```python
from build123d import *

# Parameters (mm, degrees)
F0_W     = 105.022209
F0_H     = 90.88391
F1_DEPTH = 92.202
F2_T     = -2.54
F3_W     = 99.942209
F3_H     = 87.122
F4_DEPTH = 2.794
F6_D     = 20.32
F6_DEPTH = 20.32
F7_R     = 6.310092
F8_DEPTH = 40.132


with BuildPart() as f1:
    # F0 (on Top) → F1 (new body)
    with BuildSketch(Plane.XY):
        with Locations((-23.505336, -22.022091)):
            Rectangle(F0_W, F0_H)
    extrude(amount=F1_DEPTH)

    # F2
    f2_openings = [f1.faces().sort_by_distance(p)[0] for p in [
        (-23.505337, -67.464046, 46.101),
    ]]
    offset(amount=F2_T, openings=f2_openings)

    # F3 (on face) → F4 (join)
    with BuildSketch(Plane.XZ.offset(67.464046)):
        with Locations((-23.505336, 46.101)):
            Rectangle(F3_W, F3_H)
    extrude(amount=-F4_DEPTH)

    # F6
    with Locations(Plane.XZ.offset(67.464046)):
        with Locations((-50.33106, 63.634276)):
            Hole(F6_D / 2, depth=F6_DEPTH)

    # F7 (on face) → F8 (join)
    with BuildSketch(Plane.XZ.offset(67.464046)):
        with Locations((-52.374396, 25.210666)):
            Circle(F7_R)
    extrude(amount=F8_DEPTH)


solid = f1.part
```
Source: CAD feature listing. Evaluate the final solid. Frame: model axes, mm. A direction names the side the tool comes from. Give positions to 0.01 mm unless a question says otherwise; leave off trailing zeros. Write each loop counter-clockwise with the first axis right and the second up, starting at its lowest first coordinate (ties: lowest second). Pieces come first, ordered by that corner, then holes. Notation, with made-up numbers: (38, 66.25) - (73, 66.25) arc R22 cw to (73, 89.25) - close; hole circle Ø11 at (-5, 64.25). An arc over 180 degrees is marked (long way). One line per item, written item: value. Start each with the question number.
Q1. Draft query along Z for faces 4 (the face through (-49.463, -87.249, 19.613)), 5 (the face through (-24, -21, 2.54)), 6 (the face through (-24, 23.42, 45)), 7 (the face through (-24, -64.67, 47)). Return one class per face: +Z half, -Z half, draft (parallel to the pull), parting line (faces both ways), or undercut.
Q2. Section query B-B, the plane y = -16.5. Return the cut outline in (x, z).
Q3. Set-up query: faces 1 (the face through (-73.476, -22, 45)), 2 (the face through (-48.129, -66.047, 53.716)), 3 (the face through (29.006, -23, 45)). Return all of +Z, -Z, +X, -X, +Y, -Y with unobstructed straight access to the full face (end or side cutting, diameter ignored); none if empty.
Q4. First-contact query: pin 1 Ø2 at (x, z) = (-10.5, 38.5) entering from -Y; pin 2 Ø1.5 at (x, y) = (-43, -66.5) entering from -Z; pin 3 Ø18.5 at (x, z) = (-50.33, 63.63) entering from -Y. Flat tips, straight axial feed; report the tip coordinate or a pass-through.
Q5. Material intervals for probe 1 along X at (y, z) = (-50.5, 27); probe 2 along Y at (x, z) = (-30.5, 76); probe 3 along Z at (x, y) = (-11, -16), sorted ascending. Write a range as from..to.
Q6. Section query D-D, the plane y = -93. Return the cut outline in (x, z).
Q7. Section query C-C, the plane x = -50. Return the cut outline in (y, z), then the cut area to 3 significant figures.
Q8. Section query A-A, the plane z = 80. Return the cut outline in (x, y), then the cut area to 3 significant figures.
Answer:
1. face 4: parting line
1. face 5: undercut
1. face 6: draft
1. face 7: undercut
2. outline: (-76.02, 0) - (29.01, 0) - (29.01, 92.2) - (-76.02, 92.2) - close; hole (-73.48, 2.54) - (26.47, 2.54) - (26.47, 89.66) - (-73.48, 89.66) - close
3. face 1: none
3. face 2: -Y
3. face 3: +Z, -Z, +X, +Y, -Y
4. pin 1: stops at y = -67.46
4. pin 2: stops at z = 0
4. pin 3: stops at y = 20.88
5. probe 1: x = -76.02..-73.48, 26.47..29.01
5. probe 2: y = -67.46..-64.67, 20.88..23.42
5. probe 3: z = 0..2.54, 89.66..92.2
6. outline: circle Ø12.62 at (-52.37, 25.21)
7. outline: (-107.6, 19.36) - (-67.46, 19.36) - (-67.46, 0) - (23.42, 0) - (23.42, 92.2) - (-67.46, 92.2) - (-67.46, 73.79) - (-64.67, 73.79) - (-64.67, 89.66) - (20.88, 89.66) - (20.88, 2.54) - (-64.67, 2.54) - (-64.67, 53.48) - (-67.46, 53.48) - (-67.46, 31.06) - (-107.6, 31.06) - close
7. area: 1,340 mm2
8. outline: (-76.02, -67.46) - (29.01, -67.46) - (29.01, 23.42) - (-76.02, 23.42) - close; hole (-73.48, -64.67) - (26.47, -64.67) - (26.47, 20.88) - (-73.48, 20.88) - close
8. area: 995 mm2
